Work out the finished part from the listing and answer in its coordinate system (mm). Face numbers are marked on the shaded views. Give positions to 0.01 mm unless a question says otherwise; leave off trailing zeros. Order: outer loops, then holes, each group sorted by start corner. A loop starts at its lowest first (then second) coordinate and runs counter-clockwise, first axis right, second up. Notation, with made-up numbers: M 30.25,73 L 43.25,73 A15 ccw 43.25,79 Z; hole C 74.5,-15.75 d11. An arc over 180 degrees is marked long. One line per item, written item: value.
from build123d import *

# Parameters (mm, degrees)
F1_DEPTH    = 25
F2_R        = 4
F3_DEPTH    = 17.8
F4_DEPTH    = 25
F5_T1_DEPTH = 165
F6_T1_DEPTH = 165


# Not quite as in the source:
# - a fillet or chamfer that OpenCascade refuses, or shapes differently, is made with other operations: its cross-section is extruded or revolved along the edge and cut away or added


with BuildPart() as f1:
    # F0 (on Top) → F1 (new body)
    with BuildSketch(Plane.XY):
        with BuildLine():
            ThreePointArc((4.8683269703, 74.3350517786), (8.3924837429, 75.788177233), (9.8682237508, 79.3029241619))
            Line((9.8682237508, 79.3029241619), (10.446520851, 169.3010662119))
            Line((10.446520851, 169.3010662119), (5.4466240705, 169.3331938286))
            Line((5.4466240705, 169.3331938286), (5.4466240705, 89.3331938286))
            Line((5.4466240705, 89.3331938286), (-9.5533759295, 89.3702277541))
            Line((-9.5533759295, 89.3702277541), (-54.5533759295, 89.3331938286))
            Line((-54.5533759295, 89.3331938286), (-54.5533759295, 169.3331938286))
            Line((-54.5533759295, 169.3331938286), (-59.5532727101, 169.3010662119))
            Line((-59.5532727101, 169.3010662119), (-58.9749756099, 79.3029241619))
            ThreePointArc((-58.9749756099, 79.3029241619), (-57.499235602, 75.788177233), (-53.9750788293, 74.3350517786))
            Line((-53.9750788293, 74.3350517786), (-39.5533759295, 74.3702277541))
            Line((-39.5533759295, 74.3702277541), (-9.5533759295, 74.3702277541))
            Line((-9.5533759295, 74.3702277541), (4.8683269703, 74.3350517786))
        make_face()
    extrude(amount=F1_DEPTH)

    # F2 (on face) → F3 (cut)
    with BuildSketch(Plane(origin=(-0.1816306533, 74.4662593781, 0), x_dir=(0.9999970254, 0.0024390927, 0), z_dir=(0.0024390927, -0.9999970254, 0))):
        with Locations((-24.5160218328, 12.5830201432)):
            Circle(F2_R)
    extrude(amount=-F3_DEPTH, mode=Mode.SUBTRACT)

    # F4 (cut): a face of the model
    f4_faces = [f1.faces().sort_by_distance(p)[0] for p in [
        (-24.697579561, 74.4064625271, 12.5830201432),
    ]]
    extrude(f4_faces, amount=-F4_DEPTH, mode=Mode.SUBTRACT)

    # F5: fillet of radius 15 on 1 edges, made by hand

    # F5_s2 → F5_t1 (cut)
    with BuildSketch(Plane(origin=(0.2690025781, 41.8638312931, 0), x_dir=(0, 0, 1), z_dir=(0.0064255233, 0.9999793561, 0))):
        with BuildLine():
            ThreePointArc((0, -5.6415427574), (4.3933982822, 4.9650589604), (15, 9.3584572426))
            Line((15, 9.3584572426), (0, 9.3584572426))
            Line((0, 9.3584572426), (0, -5.6415427574))
        make_face()
    extrude(amount=F5_T1_DEPTH, mode=Mode.SUBTRACT)

    # F6: fillet of radius 15 on 1 edges, made by hand

    # F6_s2 → F6_t1 (cut)
    with BuildSketch(Plane(origin=(-1.3312414161, 207.1759551176, 0), x_dir=(0, 0, 1), z_dir=(0.0064255233, -0.9999793561, 0))):
        with BuildLine():
            ThreePointArc((0, 43.4641953473), (4.3933982822, 54.0707970651), (15, 58.4641953473))
            Line((15, 58.4641953473), (0, 58.4641953473))
            Line((0, 58.4641953473), (0, 43.4641953473))
        make_face()
    extrude(amount=F6_T1_DEPTH, mode=Mode.SUBTRACT)


solid = f1.part
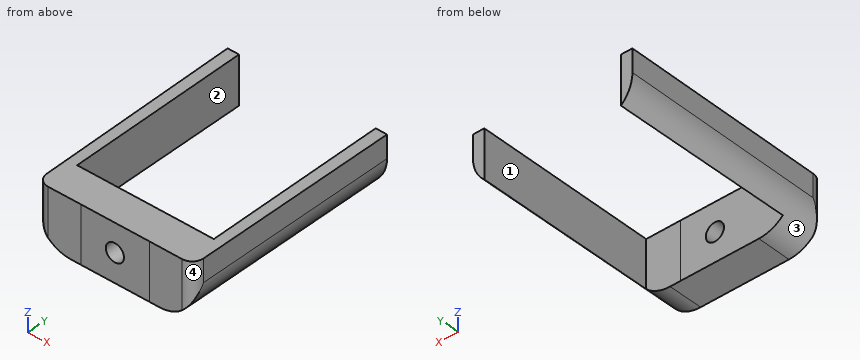
(1) Given P1, Ø5, axis at x = -7, z = 8.5, coming from the +Y side; P2, Ø2, axis at y = 126, z = 13.5, coming from the +X side; P3, Ø6, axis at y = 107, z = 13, coming from the +X side, each flat-ended and moving along its own axis, determine where each tip first touches the part or whether it passes through.
Findings:
P1: stops at y = 89.37
P2: stops at x = 10.16
P3: stops at x = 10.06
(2) Determine the mould class of the marked faces 1, 2, 3 and 4 for opening direction X: pulls with the +X half, pulls with the -X half, needs draft (parallel to the pull), parting line crosses it, or undercut.
Findings:
face 1: undercut
face 2: undercut
face 3: pulls with the -X half
face 4: pulls with the +X half
(3) Section C-C, the plane x = -37.5 is taken. Give the vertices of the cut face in (y, z), then the cut area to 3 significant figures.
Findings:
outline: M 74.37,0 L 89.35,0 L 89.35,25 L 74.37,25 Z
area: 374 mm^2
(4) Find the intervals of material crossed by probe 1 along X at (y, z) = (116, 12.25); probe 2 along Y at (x, z) = (-20, 5); probe 3 along X at (y, z) = (82, 19.5), in increasing order. Write a range as from..to.
Findings:
probe 1: x = -58.96..-54.55, 5.45..9.85
probe 2: y = 74.37..89.36
probe 3: x = -58.99..9.89
(5) Section A-A, the plane z = 21 is taken. Give the vertices of the cut face in (x, y).
Findings:
outline: M -59.55,169.3 L -58.97,79.3 A5 ccw -53.98,74.34 L -39.55,74.37 L -9.55,74.37 L 4.87,74.34 A5 ccw 9.87,79.3 L 10.45,169.3 L 5.45,169.33 L 5.45,89.33 L -9.55,89.37 L -54.55,89.33 L -54.55,169.33 Z
(6) Section B-B, the plane x = -8 is taken. Give the vertices of the cut face in (y, z), then the cut area to 3 significant figures.
Findings:
outline: M 74.37,0 L 89.37,0 L 89.37,25 L 74.37,25 Z
area: 375 mm^2
